```python
from build123d import *

# Parameters (mm, degrees)
SKETCH2_R               = 7.5
SKETCH3_R               = 8.5
SKETCH9_W               = 8.5
SKETCH9_H               = 24.609106297
CUT_EXTRUDE1_DEPTH      = 10
CUT_EXTRUDE1_DEPTH_BACK = 10
CUT_EXTRUDE2_DEPTH      = 10
CUT_EXTRUDE2_DEPTH_BACK = 10
CUT_EXTRUDE3_DEPTH      = 14
FILLET1_R               = 1
SKETCH12_R              = 1.25
CUT_EXTRUDE4_DEPTH      = 9
SKETCH13_W              = 23.915036099
SKETCH13_H              = 16.531080044
CUT_EXTRUDE5_DEPTH      = 4.5


with BuildPart() as part:
    # Sketch2 → Loft1 section 0
    with BuildSketch(Plane(origin=(0, 22, 0), x_dir=(1, 0, 0), z_dir=(0, 1, 0))):
        Circle(SKETCH2_R)
    # Sketch3 → Loft1 section 1
    with BuildSketch(Plane(origin=(0, 0, 0), x_dir=(1, 0, 0), z_dir=(0, 1, 0))):
        Circle(SKETCH3_R)
    loft()

    # Sketch9 → Cut-Extrude1 (cut, two sides)
    with BuildSketch(Plane.XY) as cut_extrude1_sk:
        with Locations((0, 23.304553149)):
            Rectangle(SKETCH9_W, SKETCH9_H)
    extrude(amount=CUT_EXTRUDE1_DEPTH, mode=Mode.SUBTRACT)
    extrude(cut_extrude1_sk.sketch, amount=-CUT_EXTRUDE1_DEPTH_BACK, mode=Mode.SUBTRACT)

    # Sketch10 → Cut-Extrude2 (cut, two sides)
    with BuildSketch(Plane(origin=(0, 0, 0), x_dir=(0, 0, -1), z_dir=(1, 0, 0))) as cut_extrude2_sk:
        with BuildLine():
            ThreePointArc((1.551397817, 22.278129211), (-3.230375863, 20.336914385), (-6.681717999, 16.5))
            Line((-6.681717999, 16.5), (-6.777720856, 11))
            Line((-6.777720856, 11), (-14.541953313, 11))
            Line((-14.541953313, 11), (-14.541953313, 25.761445422))
            Line((-14.541953313, 25.761445422), (14.965624753, 25.761445422))
            Line((14.965624753, 25.761445422), (14.965624753, 11))
            Line((14.965624753, 11), (6.777720856, 11))
            Line((6.777720856, 11), (6.043769414, 23))
            Line((6.043769414, 23), (1.551397817, 22.278129211))
        make_face()
    extrude(amount=CUT_EXTRUDE2_DEPTH, mode=Mode.SUBTRACT)
    extrude(cut_extrude2_sk.sketch, amount=-CUT_EXTRUDE2_DEPTH_BACK, mode=Mode.SUBTRACT)

    # Sketch11 → Cut-Extrude3 (cut)
    with BuildSketch(Plane(origin=(0, 0, 0), x_dir=(-1, 0, 0), z_dir=(0, -1, 0))):
        with BuildLine():
            Line((4.25, -4.5), (4.25, 4.5))
            ThreePointArc((4.25, 4.5), (0, 5.448066505), (-4.25, 4.5))
            Line((-4.25, 4.5), (-4.25, -4.5))
            ThreePointArc((-4.25, -4.5), (0, -5.448066505), (4.25, -4.5))
        make_face()
    extrude(amount=-CUT_EXTRUDE3_DEPTH, mode=Mode.SUBTRACT)

    # Fillet1
    fillet1_edges = [part.edges().sort_by_distance(p)[0] for p in [
        (4.303290893, 22, -6.104932034),
        (-4.303290893, 22, -6.104932034),
    ]]
    fillet(fillet1_edges, radius=FILLET1_R)

    # Sketch12 → Cut-Extrude4 (cut, symmetric)
    with BuildSketch(Plane(origin=(0, 0, 0), x_dir=(0, 0, -1), z_dir=(1, 0, 0))):
        with Locations((-0.5, 15.25)):
            Circle(SKETCH12_R)
    extrude(amount=CUT_EXTRUDE4_DEPTH, both=True, mode=Mode.SUBTRACT)

    # Sketch13 → Cut-Extrude5 (cut, symmetric)
    with BuildSketch(Plane(origin=(0, 0, 0), x_dir=(0, 0, -1), z_dir=(1, 0, 0))):
        with Locations((-0.392988947, 19.265540022)):
            Rectangle(SKETCH13_W, SKETCH13_H)
    extrude(amount=CUT_EXTRUDE5_DEPTH, both=True, mode=Mode.SUBTRACT)


solid = part.part
```
Can you work these out from the model? Positions are in its coordinate system, mm. A direction names the side the tool comes from. Round coordinates to 2 decimals unless told otherwise and drop trailing zeros. Loops run counter-clockwise (first coordinate to the right, second up) from the corner with the lowest first, then second, coordinate; pieces in that order, holes last.
Item 1: Will these pins go through, and if not, where does the flat tip stop? pin 1 Ø3 at (y, z) = (9.5, -2) entering from -X; pin 2 Ø3 at (y, z) = (6.5, 3) entering from +X; pin 3 Ø9 at (y, z) = (19, 3) entering from +X.
Item 2: Suppose I cut it at C-C, the plane y = 2. Write out the boundary of the cut face in (x, z), then the cut area to 3 significant figures.
Item 3: Suppose I cut it at B-B, the plane y = 15.25. Write out the boundary of the cut face in (x, z).
Item 4: Which directions (+Z, -Z, +X, -X, +Y, -Y) give clear straight access to the entire face, cutting with the end or side of a thin tool? Please do faces 5 (the flat face through (-4.5, 17, 0)), 6 (the flat face through (6, 22, -2)), 7 (the cylindrical face through (-0.061, 5.423, -5.448)).
Item 5: If we mould it in two halves opening along Y, with no side actions, what happens to faces 1 (the cylindrical face through (6.204, 14.771, -0.655)), 2 (the cylindrical face through (-5.649, 20.737, 2.619)), 3 (the cylindrical face through (-6.157, 14.771, -0.655)), 4 (the flat face through (4.5, 17, 0))? For each: +Y half, -Y half, draft (parallel to the pull), parting line (faces both ways), or undercut.
Item 6: Suppose I cut it at D-D, the plane z = 0.5. State how many separate pieces and enclosed holes the cut face has, then the cut area to 3 significant figures.
Item 7: Suppose I cut it at A-A, the plane x = 0. Write out the boundary of the cut face in (y, z), then the cut area to 3 significant figures.
Item 8: Please list where these lines run through material, in increasing order: L1, parallel to X at y = 17.25, z = -1; L2, parallel to Y at x = 0.25, z = 7.25; L3, parallel to Y at x = -7.1, z = 0.5.
Reported:
1. pin 1: stops at x = -8.07
1. pin 2: stops at x = 8.07
1. pin 3: stops at x = 7.76
2. outline: circle Ø16.82 at (0, 0); hole (-4.25, -4.5) arc R10 ccw to (4.25, -4.5) - (4.25, 4.5) arc R10 ccw to (-4.25, 4.5) - close
2. area: 135 mm2
3. outline: (-7.77, -0.75) arc R7.81 ccw to (-4.5, -6.38) - (-4.5, -0.75) - close; (-7.61, 1.75) - (-4.5, 1.75) - (-4.5, 6.38) arc R7.81 ccw to start; (4.5, -6.38) arc R7.81 ccw to (7.77, -0.75) - (4.5, -0.75) - close; (4.5, 1.75) - (7.61, 1.75) arc R7.81 ccw to (4.5, 6.38) - close
4. face 5: +Z, -Z, +Y
4. face 6: +Z, -Z, +X, -X, +Y
4. face 7: +Y, -Y
5. face 1: undercut
5. face 2: +Y half
5. face 3: undercut
5. face 4: draft
6. separate pieces: 4
6. enclosed holes: 0
6. area: 141 mm2
7. outline: (0, -8.5) - (11, -8) - (11, -5.45) - (0, -5.45) - close; (0, 5.45) - (11, 5.45) - (11, 8) - (0, 8.5) - close
7. area: 61.6 mm2
8. L1: x = -7.65 to -4.5, 4.5 to 7.65
8. L2: y = 0 to 11
8. L3: y = 0 to 14, 16.5 to 21.75
